Geometry check sheet. Reference: drawing and pictorial views, mm from the part's lowest x, y, z. A direction names the side the tool comes from. Give positions to 0.01 mm unless a question says otherwise; leave off trailing zeros. Write each loop counter-clockwise with the first axis right and the second up, starting at its lowest first coordinate (ties: lowest second). Pieces come first, ordered by that corner, then holes. Notation, with made-up numbers: (49.25, 83) - (106.25, 83) arc R28 ccw to (106.25, 101) - close; hole circle Ø8 at (-14.75, 9). An arc over 180 degrees is marked (long way). Write item = value, one per line. Start each with the question number.
(1) Section check B-B, the plane z = 3. Enter the section's corners in (x, y), plus the area to 3 significant figures.
(2) Depth check by flat-ended pin: pin 1 Ø1.8 at (x, y) = (4, 24.5) entering from -Z; pin 2 Ø2 at (y, z) = (6.5, 2.5) entering from +X; pin 3 Ø3.5 at (x, y) = (19, 15) entering from +Z. Enter the tip coordinate at first touch or a pass-through.
(3) Section check A-A, the plane y = 15. Enter the section's corners in (x, z), plus the area to 3 significant figures.
(4) Section check D-D, the plane x = 12. Enter the section's corners in (y, z), plus the area to 3 significant figures.
(5) Draft check along Y on the marked faces 5, 6 and 7. Enter one of: pulls with the +Y half, pulls with the -Y half, needs draft (parallel to the pull), parting line crosses it, or undercut.
(6) Thickness scan on L1, parallel to X at y = 15, z = 1.85; L2, parallel to Y at x = 4, z = 3.75; L3, parallel to Y at x = 4, z = 1.8. Record the ranges inside material, lowest first.
(7) Section check C-C, the plane y = 24.5. Enter the section's corners in (x, z), plus the area to 3 significant figures.
(8) Access from +Z, -Z, +X, -X, +Y, -Y to the whole of each face (thin tool, end or side, straight path). Record for the marked faces 1, 2, 3 and 4.
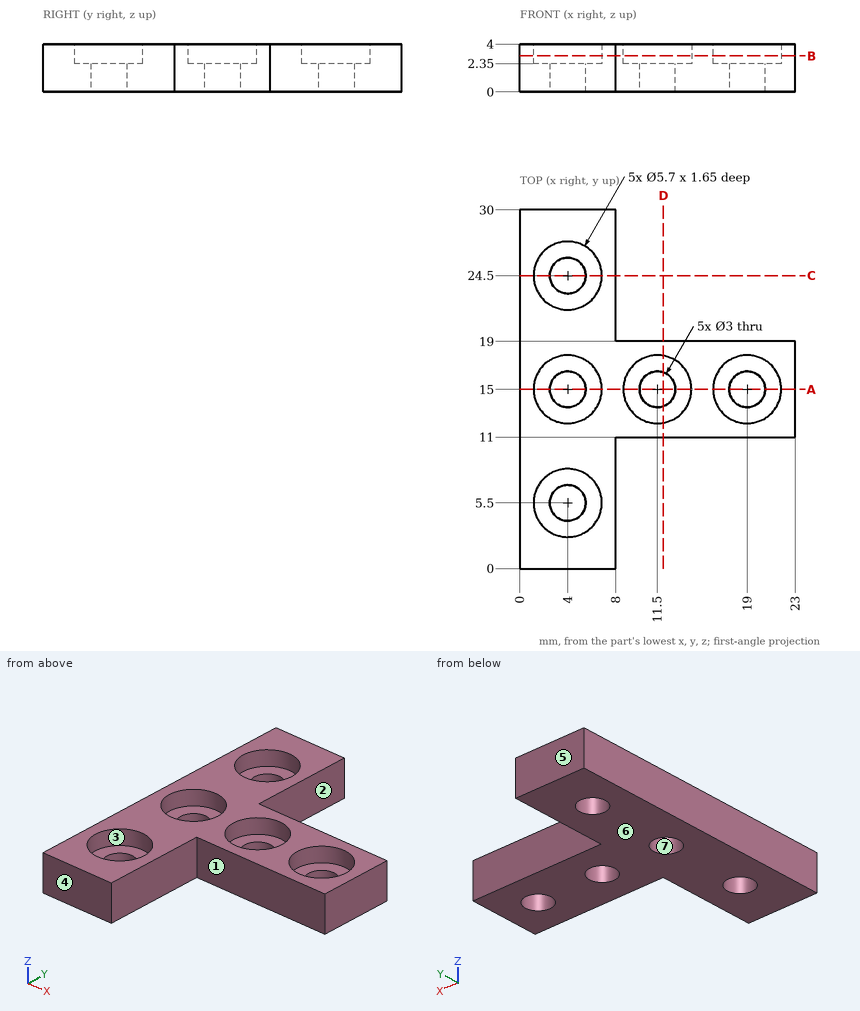
Model answer:
q1.outline = (0, 0) - (8, 0) - (8, 11) - (23, 11) - (23, 19) - (8, 19) - (8, 30) - (0, 30) - close; hole circle Ø5.7 at (4, 5.5); hole circle Ø5.7 at (4, 15); hole circle Ø5.7 at (4, 24.5); hole circle Ø5.7 at (11.5, 15); hole circle Ø5.7 at (19, 15)
q1.area = 232 mm²
q2.pin_1 = through
q2.pin_2 = 8
q2.pin_3 = 2.35
q3.outline = (0, 0) - (2.5, 0) - (2.5, 2.35) - (1.15, 2.35) - (1.15, 4) - (0, 4) - close; (5.5, 0) - (10, 0) - (10, 2.35) - (8.65, 2.35) - (8.65, 4) - (6.85, 4) - (6.85, 2.35) - (5.5, 2.35) - close; (13, 0) - (17.5, 0) - (17.5, 2.35) - (16.15, 2.35) - (16.15, 4) - (14.35, 4) - (14.35, 2.35) - (13, 2.35) - close; (20.5, 0) - (23, 0) - (23, 4) - (21.85, 4) - (21.85, 2.35) - (20.5, 2.35) - close
q3.area = 42.6 mm²
q4.outline = (11, 0) - (13.59, 0) - (13.59, 2.35) - (12.19, 2.35) - (12.19, 4) - (11, 4) - close; (16.41, 0) - (19, 0) - (19, 4) - (17.81, 4) - (17.81, 2.35) - (16.41, 2.35) - close
q4.area = 16.1 mm²
q5.face_5 = pulls with the +Y half
q5.face_6 = needs draft
q5.face_7 = undercut
q6.L1 = 0 to 2.5, 5.5 to 10, 13 to 17.5, 20.5 to 23
q6.L2 = 0 to 2.65, 8.35 to 12.15, 17.85 to 21.65, 27.35 to 30
q6.L3 = 0 to 4, 7 to 13.5, 16.5 to 23, 26 to 30
q7.outline = (0, 0) - (2.5, 0) - (2.5, 2.35) - (1.15, 2.35) - (1.15, 4) - (0, 4) - close; (5.5, 0) - (8, 0) - (8, 4) - (6.85, 4) - (6.85, 2.35) - (5.5, 2.35) - close
q7.area = 15.5 mm²
q8.face_1 = +Z, -Z, +X, -Y
q8.face_2 = +Z, -Z, +X, +Y
q8.face_3 = +Z
q8.face_4 = +Z, -Z, +X, -X, -Y
